Here's how the part is built. I have some questions about the finished solid (model axes, mm). A direction names the side the tool comes from. Coordinates: 2 decimals unless noted, no trailing zeros. Loops run counter-clockwise (first coordinate to the right, second up) from the corner with the lowest first, then second, coordinate; pieces in that order, holes last.
from build123d import *

# Parameters (mm, degrees)
F1_DEPTH = 10
F2_T     = 2
F3_DEPTH = 10


with BuildPart() as f1:
    # F0 (on Top) → F1 (new body)
    with BuildSketch(Plane.XY):
        Polygon((-4.5411753677, 10.567646683), (-9.6411753677, 10.567646683), (-9.6411753677, 5.467646683), (-7.1411753677, 2.967646683), (-9.6411753677, 0.467646683), (-9.6411753677, -4.632353317), (-4.5411753677, -4.632353317), (-2.0411753677, -2.132353317), (0.4588246323, -4.632353317), (5.5588246323, -4.632353317), (5.5588246323, 0.467646683), (3.0588246323, 2.967646683), (5.5588246323, 5.467646683), (5.5588246323, 10.567646683), (0.4588246323, 10.567646683), (-2.0411753677, 8.067646683), align=None)
        Polygon((-7.1411753677, 2.967646683), (-9.6411753677, 5.467646683), (-9.6411753677, 0.467646683), align=None)
        Polygon((-2.0411753677, -2.132353317), (-4.5411753677, -4.632353317), (0.4588246323, -4.632353317), align=None)
        Polygon((5.5588246323, 0.467646683), (5.5588246323, 5.467646683), (3.0588246323, 2.967646683), align=None)
        Polygon((0.4588246323, 10.567646683), (-4.5411753677, 10.567646683), (-2.0411753677, 8.067646683), align=None)
    extrude(amount=F1_DEPTH)

    # F2
    f2_openings = [f1.faces().sort_by_distance(p)[0] for p in [
        (-2.041175, 2.967647, 10),
    ]]
    offset(amount=F2_T, openings=f2_openings, kind=Kind.INTERSECTION)

    # F0 (on Top) → F3 (join)
    with BuildSketch(Plane.XY):
        Polygon((0.4588246323, 10.567646683), (-4.5411753677, 10.567646683), (-2.0411753677, 8.067646683), align=None)
        Polygon((5.5588246323, 0.467646683), (5.5588246323, 5.467646683), (3.0588246323, 2.967646683), align=None)
        Polygon((-7.1411753677, 2.967646683), (-9.6411753677, 5.467646683), (-9.6411753677, 0.467646683), align=None)
        Polygon((-2.0411753677, -2.132353317), (-4.5411753677, -4.632353317), (0.4588246323, -4.632353317), align=None)
    extrude(amount=F3_DEPTH)


solid = f1.part
Q1. Suppose I cut it at C-C on y = 10.25. Write out the boundary of the cut face in (x, z).
Q2. For faces 1 (the flat face through (-8.41, 1.7, 4.93)), 2 (the flat face through (-2, 12.568, 4)), which set-ups out of +Z, -Z, +X, -X, +Y, -Y let a thin tool reach every point of the face, with its end or its side?
Q3. Suppose I cut it at B-B on x = -5.25. Write out the boundary of the cut face in (y, z), and give its area (3 significant figures).
Q4. We'd pull the mould along X, two halves only. Please class faces 3 (the flat face through (-2, -6.632, 4)), 4 (the flat face through (-2, 3, 0)), 5 (the flat face through (3, -4.632, 5)), 6 (the flat face through (7.559, 3, 4)): pulls with the +X half, pulls with the -X half, needs draft (parallel to the pull), parting line crosses it, or undercut.
Q5. Please list where these lines run through material, in increasing order: probe 1 along Y at (x, z) = (4.5, 3.25); probe 2 along Y at (x, z) = (3.25, 4.5); probe 3 along X at (y, z) = (-1.75, 4.5).
Q6. Suppose I cut it at D-D on x = 4. Write out the boundary of the cut face in (y, z).
Q7. Suppose I cut it at A-A on z = 8.75. Write out the boundary of the cut face in (x, y).
Check values:
1. outline: (-11.64, -2) - (7.56, -2) - (7.56, 10) - (5.56, 10) - (5.56, 0) - (0.14, 0) - (0.14, 10) - (-4.22, 10) - (-4.22, 0) - (-9.64, 0) - (-9.64, 10) - (-11.64, 10) - close
2. face 1: +Z
2. face 2: +Z, -Z, +X, -X, +Y
3. outline: (-6.63, -2) - (12.57, -2) - (12.57, 10) - (10.57, 10) - (10.57, 0) - (-4.63, 0) - (-4.63, 10) - (-6.63, 10) - close
3. area: 78.4 mm2
4. face 3: needs draft
4. face 4: undercut
4. face 5: undercut
4. face 6: pulls with the +X half
5. probe 1: y = -6.63 to -4.63, 1.53 to 4.41, 10.57 to 12.57
5. probe 2: y = -6.63 to -4.63, 2.78 to 3.16, 10.57 to 12.57
5. probe 3: x = -11.64 to -9.64, 5.56 to 7.56
6. outline: (-6.63, -2) - (12.57, -2) - (12.57, 10) - (10.57, 10) - (10.57, 0) - (3.91, 0) - (3.91, 10) - (2.03, 10) - (2.03, 0) - (-4.63, 0) - (-4.63, 10) - (-6.63, 10) - close
7. outline: (-11.64, -6.63) - (7.56, -6.63) - (7.56, 12.57) - (-11.64, 12.57) - close; hole (-9.64, -4.63) - (-4.54, -4.63) - (-2.04, -2.13) - (0.46, -4.63) - (5.56, -4.63) - (5.56, 0.47) - (3.06, 2.97) - (5.56, 5.47) - (5.56, 10.57) - (0.46, 10.57) - (-2.04, 8.07) - (-4.54, 10.57) - (-9.64, 10.57) - (-9.64, 5.47) - (-7.14, 2.97) - (-9.64, 0.47) - close
